```python
from build123d import *

# Parameters (mm, degrees)
F0_W           = 49.7
F0_H           = 105
F0_W_2         = 33.7
F0_H_2         = 67.3
F1_DEPTH       = 2
F2_DEPTH       = 6.4
F3_DEPTH       = 4.4
F4_D           = 3.4544
F4_CSINK_D     = 7.1374
F4_CSINK_ANGLE = 82
F5_R           = 2


with BuildPart() as f1:
    # F0 (on Top) → F1 (new body)
    with BuildSketch(Plane.XY):
        Rectangle(F0_W, F0_H)
        Rectangle(F0_W_2, F0_H_2, mode=Mode.SUBTRACT)
    extrude(amount=F1_DEPTH)

    # F0 (on Top) → F2 (join)
    with BuildSketch(Plane.XY):
        Polygon((26.85, 52.5), (24.85, 52.5), (24.85, -52.5), (-24.85, -52.5), (-24.85, 52.5), (-26.85, 52.5), (-26.85, -54.5), (26.85, -54.5), align=None)
    extrude(amount=F2_DEPTH)

    # F0 (on Top) → F3 (join)
    with BuildSketch(Plane.XY):
        Polygon((-24.85, 52.5), (24.85, 52.5), (26.85, 52.5), (26.85, 54.5), (-26.85, 54.5), (-26.85, 52.5), align=None)
    extrude(amount=F3_DEPTH)

    # F4 (through all)
    with Locations(Plane(origin=(0, 0, 0), x_dir=(1, 0, 0), z_dir=(0, 0, -1))):
        with Locations((0, -48.4), (0, 48.4)):
            CounterSinkHole(F4_D / 2, F4_CSINK_D / 2, counter_sink_angle=F4_CSINK_ANGLE)

    # F5
    f5_edges = [f1.edges().sort_by_distance(p)[0] for p in [
        (26.85, 54.5, 2.2),
        (26.85, -54.5, 3.2),
        (-26.85, -54.5, 3.2),
        (-26.85, 54.5, 2.2),
    ]]
    fillet(f5_edges, radius=F5_R)


solid = f1.part
```
CAD build for the part. Positions are in the model's coordinates, mm. A direction names the side the tool comes from. Round coordinates to 2 decimals unless told otherwise and drop trailing zeros. Order: outer loops, then holes, each group sorted by start corner. A loop starts at its lowest first (then second) coordinate and runs counter-clockwise, first axis right, second up. Notation, with made-up numbers: (-20.75, 15.5) - (33.25, 15.5) arc R33 ccw to (33.25, 44.5) - close; hole circle Ø5 at (80, -39). An arc over 180 degrees is marked (long way). Use CSV: the item, a comma, the result in double quotes. Start each with the question number.
1) Two-plate mould, pull along X, no slides. Class faces 1 (the flat face through (0, 54.5, 2)), 2 (the flat face through (0, -33.65, 1)), 3 (the flat face through (-26.85, 1, 3)): pulls with the +X half, pulls with the -X half, needs draft (parallel to the pull), parting line crosses it, or undercut.
2) Tool access for faces 4 (the flat face through (0, -54.5, 3)), 5 (the flat face through (-16.85, 0, 1)), 6 (the flat face through (0, 54, 4.4)), 7 (the flat face through (0, 52.5, 3)): list every direction of +Z, -Z, +X, -X, +Y, -Y with a clear straight run to the whole face (end or side of a thin tool).
3) Saw through at A-A (x = 9). List the corners of the cut face in (y, z).
4) Pin check, flat tips, straight feed: pin 1 Ø8 at (x, y) = (-19.5, 2.5) entering from +Z; pin 2 Ø10 at (x, y) = (-18.5, -8) entering from -Z; pin 3 Ø2 at (x, y) = (9, 53.5) entering from +Z; pin 4 Ø2 at (x, z) = (-26, 6) entering from +Y. Stop position of each tip, or through.
5) Saw through at B-B (y = 0.5). List the corners of the cut face in (x, z).
6) Saw through at C-C (z = 1). List the corners of the cut face in (x, y), and give its area (3 significant figures).
7) Wall check: L1, parallel to Y at x = 0, z = 3.75; L2, parallel to X at y = -47, z = 5.5; L3, parallel to Y at x = -6.5, z = 1.75. Give the ranges that are in metal, low to high. Write a range as [from, to].
8) Saw through at D-D (y = 39.5). List the corners of the cut face in (x, z).
Values follow:
1,face 1,"needs draft"
1,face 2,"undercut"
1,face 3,"pulls with the -X half"
2,face 4,"+Z, -Z, +X, -X, -Y"
2,face 5,"+Z, -Z"
2,face 6,"+Z, +X, -X, +Y"
2,face 7,"+Z"
3,outline,"(-54.5, 0) - (-33.65, 0) - (-33.65, 2) - (-52.5, 2) - (-52.5, 6.4) - (-54.5, 6.4) - close; (33.65, 0) - (54.5, 0) - (54.5, 4.4) - (52.5, 4.4) - (52.5, 2) - (33.65, 2) - close"
4,pin 1,"stops at z = 2"
4,pin 2,"stops at z = 0"
4,pin 3,"stops at z = 4.4"
4,pin 4,"stops at y = 52.5"
5,outline,"(-26.85, 0) - (-16.85, 0) - (-16.85, 2) - (-24.85, 2) - (-24.85, 6.4) - (-26.85, 6.4) - close; (16.85, 0) - (26.85, 0) - (26.85, 6.4) - (24.85, 6.4) - (24.85, 2) - (16.85, 2) - close"
6,outline,"(-26.85, -52.5) arc R2 ccw to (-24.85, -54.5) - (24.85, -54.5) arc R2 ccw to (26.85, -52.5) - (26.85, 52.5) arc R2 ccw to (24.85, 54.5) - (-24.85, 54.5) arc R2 ccw to (-26.85, 52.5) - close; hole (-16.85, -33.65) - (16.85, -33.65) - (16.85, 33.65) - (-16.85, 33.65) - close; hole circle Ø5.4 at (0, -48.4); hole circle Ø5.4 at (0, 48.4)"
6,area,"3,540 mm2"
7,L1,"y = [-54.5, -52.5], [52.5, 54.5]"
7,L2,"x = [-26.85, -24.85], [24.85, 26.85]"
7,L3,"y = [-54.5, -33.65], [33.65, 54.5]"
8,outline,"(-26.85, 0) - (26.85, 0) - (26.85, 6.4) - (24.85, 6.4) - (24.85, 2) - (-24.85, 2) - (-24.85, 6.4) - (-26.85, 6.4) - close"
